Can you work these out from the drawing? Everything is in mm from the part's minimum corner. Coordinates: 2 decimals unless noted, no trailing zeros. Order: outer loops, then holes, each group sorted by start corner. A loop starts at its lowest first (then second) coordinate and runs counter-clockwise, first axis right, second up. Notation, with made-up numbers: M -13.5,71.25 L 14.5,71.25 A21 cw 14.5,94.25 Z; hole C 32,-17 d10. An arc over 180 degrees is marked long. Answer as a JSON object with one key per item and string values.
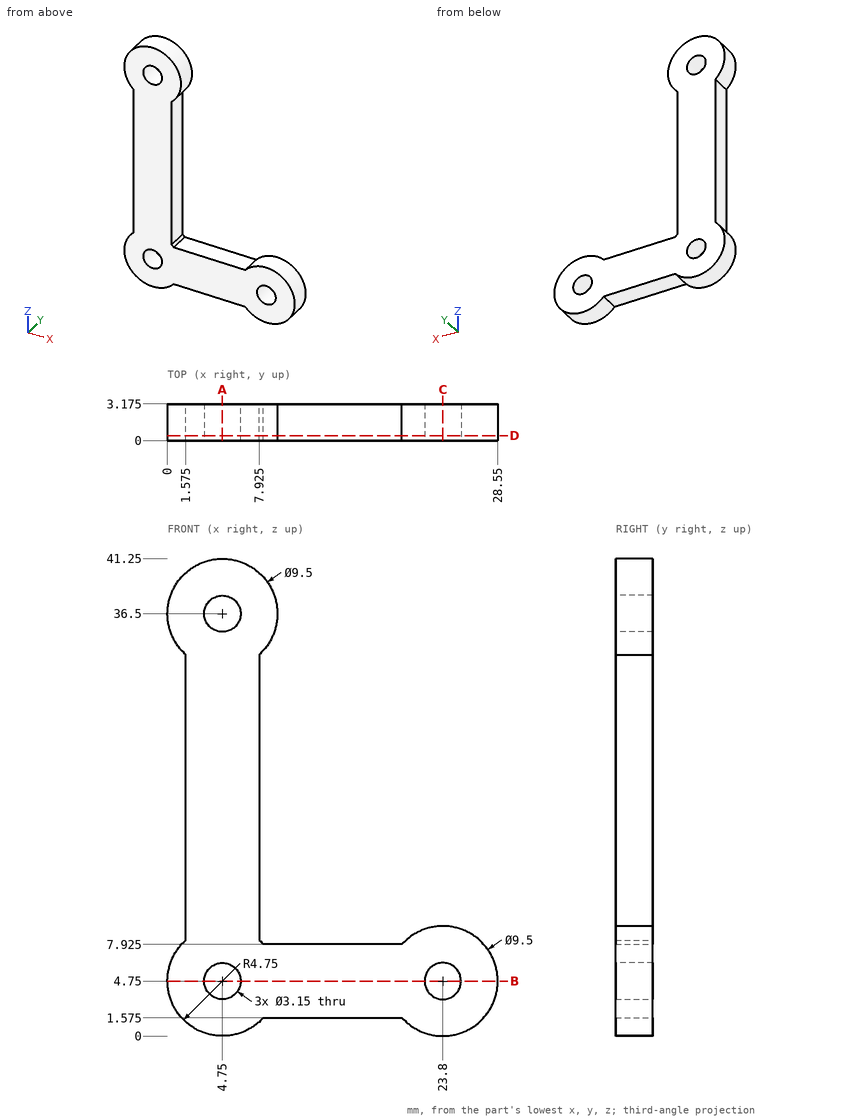
Item 1: I'm going to push flat-ended pins straight in: pin 1 (1.9 mm diameter, centred on x = 4.75, z = 36.5, fed in from +Y); pin 2 (1.5 mm diameter, centred on x = 14.5, y = 1, fed in from +Z) (3 decimals); pin 3 (1.5 mm diameter, centred on x = 9, y = 0.5, fed in from +Z). Where does each tip first touch, or does it pass through?
Answers follow:
{"pin 1": "passes through", "pin 2": "stops at z = 7.925", "pin 3": "stops at z = 39.71"}
Item 2: I want a section at A-A, the plane x = 4.75. Write out the boundary of the cut face in (y, z) (3 decimals).
Answers follow:
{"outline": "M 0,0 L 3.175,0 L 3.175,3.175 L 0,3.175 Z; M 0,6.325 L 3.175,6.325 L 3.175,34.925 L 0,34.925 Z; M 0,38.075 L 3.175,38.075 L 3.175,41.25 L 0,41.25 Z"}
Item 3: Please list where these lines run through material, in increasing order: line 1 (Z direction, x = 4.75, y = 2.3) (3 decimals); line 2 (X direction, y = 0.35, z = 31) (3 decimals).
Answers follow:
{"line 1": "z = 0 to 3.175, 6.325 to 34.925, 38.075 to 41.25", "line 2": "x = 1.575 to 7.925"}
Item 4: I want a section at C-C, the plane x = 23.8. Write out the boundary of the cut face in (y, z) (3 decimals).
Answers follow:
{"outline": "M 0,0 L 3.175,0 L 3.175,3.175 L 0,3.175 Z; M 0,6.325 L 3.175,6.325 L 3.175,9.5 L 0,9.5 Z"}
Item 5: I want a section at D-D, the plane y = 0.45. Write out the boundary of the cut face in (x, z) (3 decimals), plus the area to 3 significant figures.
Answers follow:
{"outline": "M 1.575,8.283 A4.75 ccw long 8.283,1.575 L 20.267,1.575 A4.75 ccw long 20.267,7.925 L 8.283,7.925 A4.75 ccw 7.925,8.283 L 7.925,32.967 A4.75 ccw long 1.575,32.967 Z; hole C 4.75,4.75 d3.15; hole C 4.75,36.5 d3.15; hole C 23.8,4.75 d3.15", "area": "401 mm^2"}
Item 6: I want a section at B-B, the plane z = 4.75. Write out the boundary of the cut face in (x, y) (3 decimals).
Answers follow:
{"outline": "M 0,0 L 3.175,0 L 3.175,3.175 L 0,3.175 Z; M 6.325,0 L 22.225,0 L 22.225,3.175 L 6.325,3.175 Z; M 25.375,0 L 28.55,0 L 28.55,3.175 L 25.375,3.175 Z"}
